```python
from build123d import *

# Parameters (mm, degrees)
F0_W     = 15.96
F0_H     = 7.98
F1_DEPTH = 2.94
F2_R     = 2.45
F3_DEPTH = 1.84
F4_T     = -1.57
F5_R     = 1.535
F5_R_2   = 0.765
F6_DEPTH = 1


with BuildPart() as f1:
    # F0 (on Front) → F1 (new body)
    with BuildSketch(Plane.XZ):
        with Locations((0.1376755536, 5.0412456957)):
            Rectangle(F0_W, F0_H)
    extrude(amount=F1_DEPTH)

    # F2 (on face) → F3 (join)
    with BuildSketch(Plane(origin=(0, 0, 0), x_dir=(-1, 0, 0), z_dir=(0, 1, 0))):
        with Locations((3.8373244464, 5.0412456957)):
            Circle(F2_R)
        with Locations((-4.1126755536, 5.0412456957)):
            Circle(F2_R)
    extrude(amount=F3_DEPTH)

    # F4
    f4_openings = [f1.faces().sort_by_distance(p)[0] for p in [
        (0.137676, -2.94, 5.041246),
    ]]
    offset(amount=F4_T, openings=f4_openings, kind=Kind.INTERSECTION)

    # F5 (on face) → F6 (join)
    with BuildSketch(Plane.XZ.offset(1.57)):
        with Locations((0.1626269908, 5.0662456957)):
            Circle(F5_R)
        with Locations((0.1626269908, 5.0662456957)):
            Circle(F5_R_2, mode=Mode.SUBTRACT)
    extrude(amount=F6_DEPTH)


solid = f1.part
```
The model under review builds one solid part; all positions refer to its coordinate system, in mm. A direction names the side the tool comes from. Coordinates: 2 decimals unless noted, no trailing zeros. Write each loop counter-clockwise with the first axis right and the second up, starting at its lowest first coordinate (ties: lowest second). Pieces come first, ordered by that corner, then holes. Notation, with made-up numbers: (40, -13) -> (92, -13) arc R16 cw to (92, -6) -> close; hole circle Ø3 at (-7, -12). An arc over 180 degrees is marked (long way). One line per item, written item: value. Start each with the question number.
Q1. Add section C-C, the plane y = -0.55. Give the boundary of the cut face in (x, z), then the cut area to 3 significant figures.
Q2. For faces 5 (the face through (-7.842, -1, 5)), 6 (the face through (-5.15, 0.91, 7.11)), 7 (the face through (0, -1.57, 7)), list the 3-axis set-ups (+Z, -Z, +X, -X, +Y, -Y) from which the entire face can be reached by the end or side of a thin tool; tool diameter is ignored.
Q3. The part is to be moulded in two halves that separate along X. For faces 1 (the face through (8.118, -1, 5)), 2 (the face through (0, -2, 7.461)), 3 (the face through (-4, 1.84, 5)), 4 (the face through (3.64, -0.663, 5.783)), say which applies: +X half, -X half, draft (parallel to the pull), parting line (faces both ways), or undercut.
Q4. Add section A-A, the plane y = -2. Give the boundary of the cut face in (x, z) (3 decimals).
Q5. Clearance check with flat-ended pins moving along their axes: P1, Ø1.4, axis at x = -3.84, z = 5.04, coming from the -Y side; P2, Ø0.9, axis at x = 0.16, z = 5.07, coming from the +Y side; P3, Ø4, axis at x = -2.5, z = 4, coming from the -Y side; P4, Ø3.5, axis at x = 0, z = 4.5, coming from the -Y side. State where each tip first meets the part, or that it passes through.
Q6. To check wall thickness, follow probe 1 along X at (y, z) = (-2.3, 3); probe 2 along Z at (x, y) = (2.5, -1.85); probe 3 along X at (y, z) = (-2.3, 5.5). State the ranges of each line that lie inside material, in increasing order.
Q7. Add section B-B, the plane x = 0. Give the boundary of the cut face in (y, z), then the cut area to 3 significant figures.
Response:
1. outline: (-7.84, 1.05) -> (8.12, 1.05) -> (8.12, 9.03) -> (-7.84, 9.03) -> close; hole circle Ø1.76 at (-3.84, 5.04); hole circle Ø1.76 at (4.11, 5.04)
1. area: 122 mm²
2. face 5: +Z, -Z, -X, +Y, -Y
2. face 6: +Y
2. face 7: -Y
3. face 1: +X half
3. face 2: undercut
3. face 3: draft
3. face 4: undercut
4. outline: (-7.842, 1.051) -> (8.118, 1.051) -> (8.118, 9.031) -> (-7.842, 9.031) -> close; circle Ø3.07 at (0.163, 5.066); hole (-6.272, 2.621) -> (6.548, 2.621) -> (6.548, 7.461) -> (-6.272, 7.461) -> close; hole circle Ø1.53 at (0.163, 5.066)
5. P1: y = 0.27
5. P2: y = 0
5. P3: y = -2.94
5. P4: y = -2.57
6. probe 1: -7.84 to -6.27, 6.55 to 8.12
6. probe 2: 1.05 to 2.62, 7.46 to 9.03
6. probe 3: -7.84 to -6.27, -1.31 to -0.47, 0.79 to 1.64, 6.55 to 8.12
7. outline: (-2.94, 1.05) -> (0, 1.05) -> (0, 9.03) -> (-2.94, 9.03) -> (-2.94, 7.46) -> (-1.57, 7.46) -> (-1.57, 6.59) -> (-2.57, 6.59) -> (-2.57, 5.81) -> (-1.57, 5.81) -> (-1.57, 4.32) -> (-2.57, 4.32) -> (-2.57, 3.54) -> (-1.57, 3.54) -> (-1.57, 2.62) -> (-2.94, 2.62) -> close
7. area: 18.4 mm²
